from build123d import *

# Parameters (mm, degrees)
F0_W     = 60
F0_H     = 60
F1_DEPTH = 5
F2_W     = 50
F2_H     = 50
F3_DEPTH = 5
F4_W     = 20
F4_H     = 40
F5_DEPTH = 10


with BuildPart() as f1:
    # F0 (on Top) → F1 (new body)
    with BuildSketch(Plane.XY):
        with Locations((-21.16647, 5.48928)):
            Rectangle(F0_W, F0_H)
    extrude(amount=F1_DEPTH)

    # F2 (on face) → F3 (join)
    with BuildSketch(Plane(origin=(0, 0, 0), x_dir=(1, 0, 0), z_dir=(0, 0, -1))):
        with Locations((-21.16647, -5.48928)):
            Rectangle(F2_W, F2_H)
    extrude(amount=F3_DEPTH)

    # F4 (on face) → F5 (cut)
    with BuildSketch(Plane.XY.offset(5)):
        with Locations((-21.16647, 6.135008)):
            Rectangle(F4_W, F4_H)
    extrude(amount=-F5_DEPTH, mode=Mode.SUBTRACT)


solid = f1.part
Could you check a few things on this model? Use its own coordinates, in mm. A direction names the side the tool comes from. Give positions to 0.01 mm unless a question says otherwise; leave off trailing zeros. Order: outer loops, then holes, each group sorted by start corner. A loop starts at its lowest first (then second) coordinate and runs counter-clockwise, first axis right, second up.
1. Suppose I cut it at A-A (z = 1). Write out the boundary of the cut face in (x, y) (3 decimals), plus the area to 3 significant figures.
Answers below:
outline: (-51.166, -24.511) - (8.834, -24.511) - (8.834, 35.489) - (-51.166, 35.489) - close; hole (-31.166, -13.865) - (-11.166, -13.865) - (-11.166, 26.135) - (-31.166, 26.135) - close
area: 2,800 mm2
2. For pin 1 (2.5 mm diameter, centred on x = -16.5, z = -3, fed in from +Y); pin 2 (2.5 mm diameter, centred on y = 1.5, z = -2.5, fed in from -X); pin 3 (1.5 mm diameter, centred on x = -9, z = -2.5, fed in from -Y), each with a flat end and sliding along its axis, tell me the tip position at first contact or that it passes through.
Answers below:
pin 1: stops at y = 30.49
pin 2: stops at x = -46.17
pin 3: stops at y = -19.51
3. Thinking about a two-plate mould opening in X: for faces 1 (the flat face through (-31.166, 6, 0)), 2 (the flat face through (-33, 5, -5)), 3 (the flat face through (-46.166, 6, -2)), which applies, +X half, -X half, draft (parallel to the pull), parting line (faces both ways), or undercut?
Answers below:
face 1: undercut
face 2: draft
face 3: -X half
4. Suppose I cut it at C-C (x = -25). Write out the boundary of the cut face in (y, z) (3 decimals).
Answers below:
outline: (-24.511, 0) - (-19.511, 0) - (-19.511, -5) - (-13.865, -5) - (-13.865, 5) - (-24.511, 5) - close; (26.135, -5) - (30.489, -5) - (30.489, 0) - (35.489, 0) - (35.489, 5) - (26.135, 5) - close
5. Suppose I cut it at D-D (x = 1.5). Write out the boundary of the cut face in (y, z), plus the area to 3 significant figures.
Answers below:
outline: (-24.51, 0) - (-19.51, 0) - (-19.51, -5) - (30.49, -5) - (30.49, 0) - (35.49, 0) - (35.49, 5) - (-24.51, 5) - close
area: 550 mm2
6. Which directions (+Z, -Z, +X, -X, +Y, -Y) give clear straight access to the entire face, cutting with the end or side of a thin tool? Please do faces 4 (the flat face through (-21, -13.865, 0)), 5 (the flat face through (-22, -19.511, -2)), 6 (the flat face through (-22, 30.489, -2)).
Answers below:
face 4: +Z, -Z
face 5: -Z, +X, -X, -Y
face 6: -Z, +X, -X, +Y
7. I need wall thicknesses on L1, parallel to X at y = -11.5, z = -1; L2, parallel to X at y = 10.5, z = 2.75; L3, parallel to Y at x = -26.5, z = 0.5 (3 decimals). Which ranges of each line are inside material? Lowest first, please.
Answers below:
L1: x = -46.17 to -31.17, -11.17 to 3.83
L2: x = -51.17 to -31.17, -11.17 to 8.83
L3: y = -24.511 to -13.865, 26.135 to 35.489
8. Suppose I cut it at B-B (y = 22). Write out the boundary of the cut face in (x, z), plus the area to 3 significant figures.
Answers below:
outline: (-51.17, 0) - (-46.17, 0) - (-46.17, -5) - (-31.17, -5) - (-31.17, 5) - (-51.17, 5) - close; (-11.17, -5) - (3.83, -5) - (3.83, 0) - (8.83, 0) - (8.83, 5) - (-11.17, 5) - close
area: 350 mm2
